Check sheet for the modelled part. Datum: model origin and axes. Units: mm. Round coordinates to 2 decimals unless told otherwise and drop trailing zeros. Write each loop counter-clockwise with the first axis right and the second up, starting at its lowest first coordinate (ties: lowest second). Pieces come first, ordered by that corner, then holes.
Item 1: Material ranges on line 1 along Y through (x, z) = (-23, 1.4); line 2 along X through (y, z) = (150, 0.85); line 3 along X through (y, z) = (151, 3), recorded low to high.
Item 2: Section check C-C, the plane x = -45. Record the cut outline in (y, z), plus the area to 3 significant figures.
Item 3: Section check B-B, the plane y = 16. Record the cut outline in (x, z), plus the area to 3 significant figures.
Item 4: Depth check by flat-ended pin: pin 1 (4 mm diameter, centred on x = -23, y = 150, fed in from +Z); pin 2 (10 mm diameter, centred on x = 53, y = -15, fed in from -Z); pin 3 (1 mm diameter, centred on y = 75, z = 2.5, fed in from -X); pin 4 (2 mm diameter, centred on x = -222, z = 1.5, fed in from +Y). Enter the tip coordinate at first touch or a pass-through.
Item 5: Section check A-A, the plane z = 0.95. State how many separate pieces and enclosed holes the cut face has, plus the area to 3 significant figures.
Item 6: Release check for a two-part mould opening along X. For faces 1 (the flat face through (68.856, 82.575, 1.972)), 2 (the cylindrical face through (-50.461, -16.947, 1.972)), 3 (the flat face through (-46, 49, 4)), 4 (the flat face through (-150.574, 86.43, 1.972)) record: pulls with the +X half, pulls with the -X half, needs draft (parallel to the pull), parting line crosses it, or undercut.
from build123d import *

# Parameters (mm, degrees)
BOSS_EXTRUDE1_DEPTH      = 4
M5_CLEARANCE_HOLE1_D     = 5.3
FILLET1_R                = 5
M6_CLEARANCE_HOLE1_D     = 6.4
M6_CLEARANCE_HOLE1_DEPTH = 8
M6_CLEARANCE_HOLE1_TIP   = 1.922753981


with BuildPart() as part:
    # Sketch1 → Boss-Extrude1 (new body)
    with BuildSketch(Plane.XY):
        Polygon((-267, -30), (98, -30), (98, 0), (38, 170), (-38, 170), (-267, 0), align=None)
    extrude(amount=BOSS_EXTRUDE1_DEPTH)

    # M5 Clearance Hole1 (through all)
    with Locations(Plane.XY.offset(4)):
        with Locations((-23, 150), (-23, 67.5), (-23, -15), (23, -15), (23, 150), (23, 67.5), (-83, -15), (83, -15), (-222, -15)):
            Hole(M5_CLEARANCE_HOLE1_D / 2)

    # Fillet1
    fillet1_edges = [part.edges().sort_by_distance(p)[0] for p in [
        (-267, 0, 2),
        (-38, 170, 2),
        (38, 170, 2),
        (98, 0, 2),
        (98, -30, 2),
        (-267, -30, 2),
    ]]
    fillet(fillet1_edges, radius=FILLET1_R)

    # M6 Clearance Hole1
    with Locations(Plane.XY.offset(4)):
        with Locations((-252, -15), (-53, -15), (53, -15)):
            Hole(M6_CLEARANCE_HOLE1_D / 2, depth=M6_CLEARANCE_HOLE1_DEPTH)
            with Locations((0, 0, -(M6_CLEARANCE_HOLE1_DEPTH + M6_CLEARANCE_HOLE1_TIP / 2))):  # 118° drill point
                Cone(0, M6_CLEARANCE_HOLE1_D / 2, M6_CLEARANCE_HOLE1_TIP, mode=Mode.SUBTRACT)


solid = part.part
Values found:
1. line 1: y = -30 to -17.65, -12.35 to 64.85, 70.15 to 147.35, 152.65 to 170
1. line 2: x = -64.94 to -25.65, -20.35 to 20.35, 25.65 to 45.06
1. line 3: x = -63.59 to -25.45, -20.55 to 20.55, 25.45 to 44.71
2. outline: (-30, 0) - (164.8, 0) - (164.8, 4) - (-30, 4) - close
2. area: 779 mm2
3. outline: (-245.45, 0) - (92.35, 0) - (92.35, 4) - (-245.45, 4) - close
3. area: 1,350 mm2
4. pin 1: passes through
4. pin 2: stops at z = 0
4. pin 3: stops at x = -166.64
4. pin 4: stops at y = 34.15
5. separate pieces: 1
5. enclosed holes: 12
5. area: 48,100 mm2
6. face 1: pulls with the +X half
6. face 2: undercut
6. face 3: needs draft
6. face 4: pulls with the -X half
